The listing builds one solid part. Answer for the finished solid, in the listing's coordinates (mm). Face numbers are marked on the shaded views. Give positions to 0.01 mm unless a question says otherwise; leave off trailing zeros. Write each loop counter-clockwise with the first axis right and the second up, starting at its lowest first coordinate (ties: lowest second). Pieces come first, ordered by that corner, then holes. Notation, with made-up numbers: M 79.5,10 L 122.5,10 A27 ccw 122.5,44 Z; hole C 50.5,55 d10. An arc over 180 degrees is marked long. Return JSON: item names as keys, results as strings.
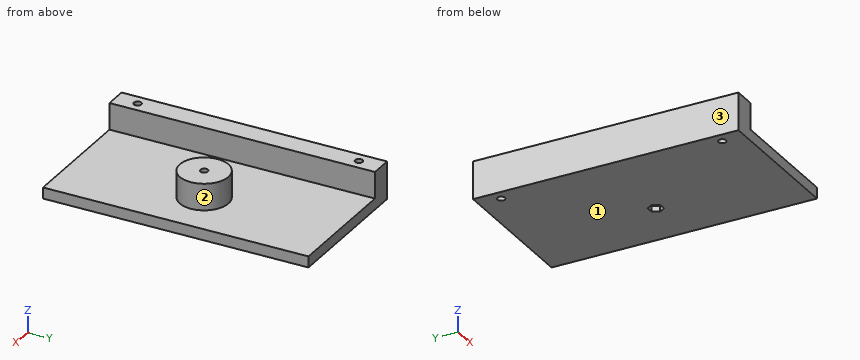
from build123d import *

# Parameters (mm, degrees)
SKETCH1_W           = 120
SKETCH1_H           = 65
BOSS_EXTRUDE1_DEPTH = 5
SKETCH2_W           = 10
SKETCH2_H           = 120
BOSS_EXTRUDE2_DEPTH = 12
SKETCH3_R           = 11
BOSS_EXTRUDE3_DEPTH = 12
SKETCH4_R           = 1.7
CUT_EXTRUDE1_DEPTH  = 22
SKETCH5_R           = 1.7
CUT_EXTRUDE2_DEPTH  = 17
CUT_EXTRUDE3_DEPTH  = 2.6


with BuildPart() as part:
    # Sketch1 → Boss-Extrude1 (new body)
    with BuildSketch(Plane(origin=(0, 0, 0), x_dir=(0, 1, 0), z_dir=(0, 0, 1))):
        Rectangle(SKETCH1_W, SKETCH1_H)
    extrude(amount=BOSS_EXTRUDE1_DEPTH)

    # Sketch2 → Boss-Extrude2 (add)
    with BuildSketch(Plane.XY.offset(5)):
        with Locations((-27.5, 0)):
            Rectangle(SKETCH2_W, SKETCH2_H)
    extrude(amount=BOSS_EXTRUDE2_DEPTH)

    # Sketch3 → Boss-Extrude3 (add)
    with BuildSketch(Plane.XY.offset(5)):
        with Locations((8.99, 0)):
            Circle(SKETCH3_R)
    extrude(amount=BOSS_EXTRUDE3_DEPTH)

    # Sketch4 → Cut-Extrude1 (cut)
    with BuildSketch(Plane.XY.offset(17)):
        with Locations((-27.5, 50)):
            Circle(SKETCH4_R)
        with Locations((-27.5, -50)):
            Circle(SKETCH4_R)
    extrude(amount=-CUT_EXTRUDE1_DEPTH, mode=Mode.SUBTRACT)

    # Sketch5 → Cut-Extrude2 (cut)
    with BuildSketch(Plane.XY.offset(17)):
        with Locations((8.99, 0)):
            Circle(SKETCH5_R)
    extrude(amount=-CUT_EXTRUDE2_DEPTH, mode=Mode.SUBTRACT)

    # Sketch6 → Cut-Extrude3 (cut)
    with BuildSketch(Plane(origin=(0, 0, 0), x_dir=(1, 0, 0), z_dir=(0, 0, -1))):
        Polygon((7.383808361, -2.87230716), (10.674395148, -2.827156342), (12.280586787, 0.045150817), (10.596191639, 2.87230716), (7.305604852, 2.827156342), (5.699413213, -0.045150817), align=None)
    extrude(amount=-CUT_EXTRUDE3_DEPTH, mode=Mode.SUBTRACT)


solid = part.part
Item 1: Determine the mould class of the marked faces 1, 2 and 3 for opening direction X: +X half, -X half, draft (parallel to the pull), parting line (faces both ways), or undercut.
Geometry results:
{"face 1": "draft", "face 2": "undercut", "face 3": "-X half"}
Item 2: A cutting plane is placed at B-B, the plane y = 50. Write down the section's boundary in (x, z), plus the area to 3 significant figures.
Geometry results:
{"outline": "M -32.5,0 L -29.2,0 L -29.2,17 L -32.5,17 Z; M -25.8,0 L 32.5,0 L 32.5,5 L -22.5,5 L -22.5,17 L -25.8,17 Z", "area": "387 mm2"}
Item 3: A cutting plane is placed at C-C, the plane x = -27.5. Write down the section's boundary in (y, z).
Geometry results:
{"outline": "M -60,0 L -51.7,0 L -51.7,17 L -60,17 Z; M -48.3,0 L 48.3,0 L 48.3,17 L -48.3,17 Z; M 51.7,0 L 60,0 L 60,17 L 51.7,17 Z"}
Item 4: Given pin 1 Ø4.5 at (x, y) = (8.99, 0) entering from -Z; pin 2 Ø2 at (y, z) = (27, 12) entering from +X; pin 3 Ø5 at (x, z) = (5.5, 11.5) entering from +Y, each flat-ended and moving along its own axis, determine where each tip first touches the part or whether it passes through.
Geometry results:
{"pin 1": "stops at z = 2.6", "pin 2": "stops at x = -22.5", "pin 3": "stops at y = 10.96"}
Item 5: Find the intervals of material crossed by line 1 (Y direction, x = -27.5, z = 9); line 2 (Y direction, x = -26.5, z = 11.75); line 3 (Z direction, x = -10, y = -19.5), in increasing order.
Geometry results:
{"line 1": "y = -60 to -51.7, -48.3 to 48.3, 51.7 to 60", "line 2": "y = -60 to -51.37, -48.63 to 48.63, 51.37 to 60", "line 3": "z = 0 to 5"}
Item 6: A cutting plane is placed at D-D, the plane y = 34. Write down the section's boundary in (x, z), plus the area to 3 significant figures.
Geometry results:
{"outline": "M -32.5,0 L 32.5,0 L 32.5,5 L -22.5,5 L -22.5,17 L -32.5,17 Z", "area": "445 mm2"}
Item 7: A cutting plane is placed at A-A, the plane z = 7.5. Write down the section's boundary in (x, y).
Geometry results:
{"outline": "M -32.5,-60 L -22.5,-60 L -22.5,60 L -32.5,60 Z; C 8.99,0 d22; hole C -27.5,-50 d3.4; hole C -27.5,50 d3.4; hole C 8.99,0 d3.4"}
